Could you check a few things on this model? Use its own coordinates, in mm. Face numbers are marked on the shaded views. Coordinates: 2 decimals unless noted, no trailing zeros. Order: outer loops, then holes, each group sorted by start corner. A loop starts at its lowest first (then second) coordinate and runs counter-clockwise, first axis right, second up. Notation, with made-up numbers: (20, 43.25) - (54, 43.25) arc R21 ccw to (54, 73.25) - close; hole circle Ø5 at (-5.5, 16). An arc over 180 degrees is marked (long way). Answer as CSV lines item,"result". Start each with the question number.
1. I want a section at A-A, the plane x = -2.8. List the corners of the cut face in (y, z) for me.
2. I need wall thicknesses on probe 1 along Z at (x, y) = (-2.8, 1); probe 2 along X at (y, z) = (1.2, 0); probe 3 along Z at (x, y) = (-2, 2.15). Which ranges of each line are inside material? Lowest first, please.
3. I want a section at C-C, the plane z = 0. List the corners of the cut face in (x, y) for me.
4. I want a section at B-B, the plane y = 1.15. List the corners of the cut face in (x, z) for me, and give its area (3 significant figures).
5. Thinking about a two-plate mould opening in Z: for the marked faces 1, 2 and 3, which applies, released by +Z, released by -Z, zero draft, split by the parting line, or undercut?
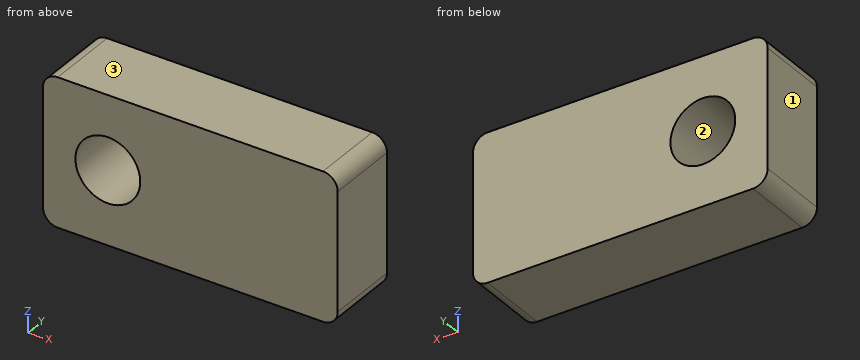
from build123d import *

# Parameters (mm, degrees)
SKETCH1_W           = 10
SKETCH1_H           = 5
SKETCH1_R           = 1.1
BOSS_EXTRUDE1_DEPTH = 2.5
FILLET1_R           = 0.5


with BuildPart() as part:
    # Sketch1 → Boss-Extrude1 (new body)
    with BuildSketch(Plane(origin=(0, 0, 0), x_dir=(1, 0, 0), z_dir=(0, 1, 0))):
        Rectangle(SKETCH1_W, SKETCH1_H)
        with Locations((-2.8, 0)):
            Circle(SKETCH1_R, mode=Mode.SUBTRACT)
    extrude(amount=BOSS_EXTRUDE1_DEPTH)

    # Fillet1
    fillet1_edges = [part.edges().sort_by_distance(p)[0] for p in [
        (5, 1.25, 2.5),
        (-5, 1.25, 2.5),
        (-5, 1.25, -2.5),
        (5, 1.25, -2.5),
    ]]
    fillet(fillet1_edges, radius=FILLET1_R)


solid = part.part
Solved:
1,outline,"(0, -2.5) - (2.5, -2.5) - (2.5, -1.1) - (0, -1.1) - close; (0, 1.1) - (2.5, 1.1) - (2.5, 2.5) - (0, 2.5) - close"
2,probe 1,"z = -2.5 to -1.1, 1.1 to 2.5"
2,probe 2,"x = -5 to -3.9, -1.7 to 5"
2,probe 3,"z = -2.5 to -0.75, 0.75 to 2.5"
3,outline,"(-5, 0) - (-3.9, 0) - (-3.9, 2.5) - (-5, 2.5) - close; (-1.7, 0) - (5, 0) - (5, 2.5) - (-1.7, 2.5) - close"
4,outline,"(-5, -2) arc R0.5 ccw to (-4.5, -2.5) - (4.5, -2.5) arc R0.5 ccw to (5, -2) - (5, 2) arc R0.5 ccw to (4.5, 2.5) - (-4.5, 2.5) arc R0.5 ccw to (-5, 2) - close; hole circle Ø2.2 at (-2.8, 0)"
4,area,"46.0 mm2"
5,face 1,"zero draft"
5,face 2,"undercut"
5,face 3,"released by +Z"
